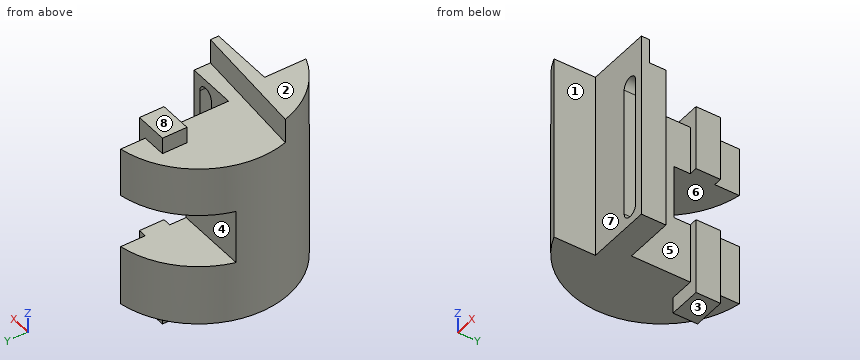
```python
from build123d import *

# Parameters (mm, degrees)
BOSS_EXTRUDE1_DEPTH      = 115
CUT_EXTRUDE1_START       = -15
CUT_EXTRUDE1_DEPTH       = 15
BOSS_EXTRUDE2_DEPTH      = 10
BOSS_EXTRUDE2_DEPTH_BACK = 110
SKETCH3_W                = 20
SKETCH3_H                = 15
CUT_EXTRUDE2_DEPTH       = 148.83859442
CUT_EXTRUDE2_DEPTH_BACK  = 148.83859442
SKETCH4_W                = 33
SKETCH4_H                = 40
CUT_EXTRUDE3_DEPTH       = 153.581945197
CUT_EXTRUDE3_DEPTH_BACK  = 153.581945197


with BuildPart() as part:
    # Sketch1 → Boss-Extrude1 (new body)
    with BuildSketch(Plane.XY):
        with BuildLine():
            Line((0, 0), (-40, 0))
            Line((-40, 0), (-40, -25.362796982))
            ThreePointArc((-40, -25.362796982), (-75.256322222, 31.603413808), (-30, 81))
            Line((-30, 81), (-30, 15))
            Line((-30, 15), (0, 15))
            Line((0, 15), (0, 0))
        make_face()
    extrude(amount=BOSS_EXTRUDE1_DEPTH)

    # Sketch2 → Cut-Extrude1 (cut)
    with BuildSketch(Plane.XY.offset(115).offset(CUT_EXTRUDE1_START)):
        with BuildLine():
            Line((0, 5), (-73.226382592, 10.685668923))
            ThreePointArc((-73.226382592, 10.685668923), (-67.28023004, 55.474290815), (-30, 81))
            Line((-30, 81), (-30, 15))
            Line((-30, 15), (0, 15))
            Line((0, 15), (0, 5))
        make_face()
    extrude(amount=CUT_EXTRUDE1_DEPTH, mode=Mode.SUBTRACT)

    # Sketch3 → Boss-Extrude2 (add, two sides: drawn at the far end of the back side and taken through both)
    with BuildSketch(Plane(origin=(0, 0, 0), x_dir=(-1, 0, 0), z_dir=(0, 0, -1)).offset(-BOSS_EXTRUDE2_DEPTH_BACK)):
        with Locations((35, 58.5)):
            Rectangle(SKETCH3_W, SKETCH3_H)
    extrude(amount=BOSS_EXTRUDE2_DEPTH + BOSS_EXTRUDE2_DEPTH_BACK)

    # Sketch4 → Cut-Extrude2 (cut, two sides: drawn at the far end of the back side and taken through both)
    with BuildSketch(Plane(origin=(-30, 0, 0), x_dir=(0, 0, -1), z_dir=(1, 0, 0)).offset(-CUT_EXTRUDE2_DEPTH_BACK)):
        with Locations((-53.5, 61)):
            Rectangle(SKETCH4_W, SKETCH4_H)
    extrude(amount=CUT_EXTRUDE2_DEPTH + CUT_EXTRUDE2_DEPTH_BACK, mode=Mode.SUBTRACT)

    # Sketch5 → Cut-Extrude3 (cut, two sides: drawn at the far end of the back side and taken through both)
    with BuildSketch(Plane(origin=(0, 15, 0), x_dir=(1, 0, 0), z_dir=(0, 1, 0)).offset(-CUT_EXTRUDE3_DEPTH_BACK)):
        with BuildLine():
            Line((-4.98034548, -10), (-4.98034548, -90))
            ThreePointArc((-4.98034548, -90), (-9.98034548, -95), (-14.98034548, -90))
            Line((-14.98034548, -90), (-14.98034548, -10))
            ThreePointArc((-14.98034548, -10), (-9.98034548, -5), (-4.98034548, -10))
        make_face()
    extrude(amount=CUT_EXTRUDE3_DEPTH + CUT_EXTRUDE3_DEPTH_BACK, mode=Mode.SUBTRACT)


solid = part.part
```
Geometry check sheet. Reference: the model listing, model coordinates, mm. Face numbers are marked on the shaded views. A direction names the side the tool comes from. Coordinates: 2 decimals unless noted, no trailing zeros. Loops run counter-clockwise (first coordinate to the right, second up) from the corner with the lowest first, then second, coordinate; pieces in that order, holes last.
Item 1: Sectioned sample at D-D, the plane x = -32. Record the boundary of the cut face in (y, z).
Item 2: Release check for a two-part mould opening along Z. For the marked faces 1, 2, 3 and 4 record: released by +Z, released by -Z, zero draft, split by the parting line, or undercut.
Item 3: Sectioned sample at B-B, the plane x = -11. Record the boundary of the cut face in (y, z).
Item 4: Access from +Z, -Z, +X, -X, +Y, -Y to the whole of each face (thin tool, end or side, straight path). Record for the marked faces 5, 6, 7 and 8.
Item 5: Sectioned sample at A-A, the plane z = 44. Record the boundary of the cut face in (x, y), then the cut area to 3 significant figures.
Item 6: Go/stop test with flat-tipped pins: pin 1 Ø3 at (y, z) = (61.5, -7.5) entering from -X; pin 2 Ø22 at (x, z) = (-38.5, 80.5) entering from -Y; pin 3 Ø16.5 at (y, z) = (58.5, 83) entering from +X; pin 4 Ø3 at (x, y) = (-23.5, 68) entering from -Z. Record where each tip stops, or that it passes through.
Item 7: Thickness scan on line 1 (Z direction, x = -61, y = 53.5); line 2 (Z direction, x = -36.5, y = 52.5); line 3 (X direction, y = 24.5, z = 45). Record the ranges inside material, lowest first.
Item 8: Sectioned sample at C-C, the plane z = 87.5. Record the boundary of the cut face in (x, y), then the cut area to 3 significant figures.
Check result:
1. outline: (0, 0) - (51, 0) - (51, -10) - (66, -10) - (66, 0) - (80.6, 0) - (80.6, 37) - (41, 37) - (41, 70) - (80.6, 70) - (80.6, 100) - (66, 100) - (66, 110) - (51, 110) - (51, 100) - (7.48, 100) - (7.48, 115) - (0, 115) - close
2. face 1: zero draft
2. face 2: released by +Z
2. face 3: released by -Z
2. face 4: undercut
3. outline: (0, 0) - (15, 0) - (15, 5.11) - (0, 5.11) - close; (0, 94.89) - (15, 94.89) - (15, 100) - (5.85, 100) - (5.85, 115) - (0, 115) - close
4. face 5: +Z, -Z, +X
4. face 6: +X, -X, +Y
4. face 7: +Z, -Z, +X, -Y
4. face 8: +Z, +X, -X, +Y
5. outline: (-73.55, 41) arc R55.5 ccw to (-40, -25.36) - (-40, 0) - (-14.98, 0) - (-14.98, 15) - (-30, 15) - (-30, 41) - close; (-4.98, 0) - (0, 0) - (0, 15) - (-4.98, 15) - close
5. area: 2,550 mm2
6. pin 1: stops at x = -45
6. pin 2: stops at y = -25.36
6. pin 3: stops at x = -25
6. pin 4: passes through
7. line 1: z = 0 to 37, 70 to 100
7. line 2: z = -10 to 37, 70 to 110
7. line 3: x = -75.47 to -30
8. outline: (-40, -25.36) - (-40, 0) - (-14.98, 0) - (-14.98, 15) - (-30, 15) - (-30, 51) - (-25, 51) - (-25, 66) - (-30, 66) - (-30, 81) arc R55.5 ccw to start; (-4.98, 0) - (0, 0) - (0, 15) - (-4.98, 15) - close
8. area: 3,840 mm2
